The model under review builds one solid part; all positions refer to its coordinate system, in mm. Give positions to 0.01 mm unless a question says otherwise; leave off trailing zeros. Loops run counter-clockwise (first coordinate to the right, second up) from the corner with the lowest first, then second, coordinate; pieces in that order, holes last. Notation, with made-up numbers: M -30.75,0 L -11.75,0 A21 ccw -11.75,8 Z; hole C 18.5,77 d1. An arc over 180 degrees is marked long. Return JSON: item names as keys, results as strings.
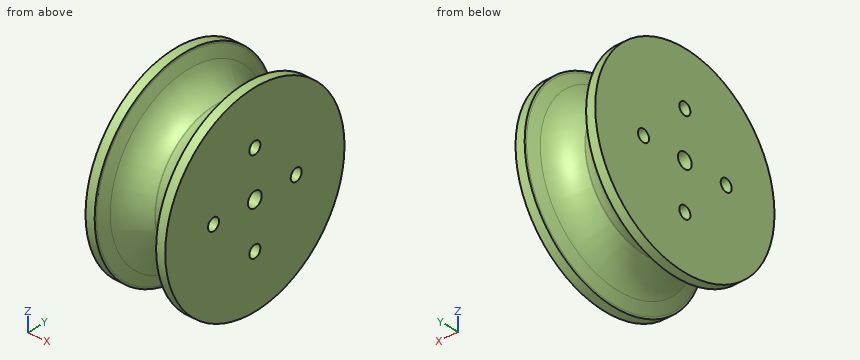
```python
from build123d import *

# Parameters (mm, degrees)
SKETCH1_W          = 3
SKETCH1_H          = 30
SKETCH2_R          = 2
CUT_EXTRUDE1_DEPTH = 31


with BuildPart() as part:
    # Sketch1 → Revolve1 (revolve)
    with BuildSketch(Plane.XY):
        with BuildLine():
            ThreePointArc((0.101961368, 31.893841841), (0, 31.900056883), (-0.101961368, 31.893841841))
            ThreePointArc((-0.101961368, 31.893841841), (-5.309821172, 29.73045951), (-8.646594366, 25.184255434))
            Line((-8.646594366, 25.184255434), (-9.965363022, 21.693397226))
            ThreePointArc((-9.965363022, 21.693397226), (-10.046395323, 21.401631123), (-10.073702174, 21.100055213))
            Line((-10.073702174, 21.100055213), (-10.073702174, 51.100055213))
            Line((-10.073702174, 51.100055213), (10.073702174, 51.100055213))
            Line((10.073702174, 51.100055213), (10.073702174, 21.100055213))
            ThreePointArc((10.073702174, 21.100055213), (10.046395323, 21.401631123), (9.965363022, 21.693397226))
            Line((9.965363022, 21.693397226), (8.646594366, 25.184255434))
            ThreePointArc((8.646594366, 25.184255434), (5.309821172, 29.73045951), (0.101961368, 31.893841841))
        make_face()
        with Locations((-11.573702174, 36.100055213)):
            Rectangle(SKETCH1_W, SKETCH1_H)
        with Locations((11.573702174, 36.100055213)):
            Rectangle(SKETCH1_W, SKETCH1_H)
    revolve(axis=Axis((-31.343058989, 53.600055213, 0), (1, 0, 0)))

    # Sketch2 → Cut-Extrude1 (cut)
    with BuildSketch(Plane.ZY.offset(13.073702174)):
        with Locations((0, 68.600055213)):
            Circle(SKETCH2_R)
        with Locations((15, 53.600055213)):
            Circle(SKETCH2_R)
        with Locations((0, 38.600055213)):
            Circle(SKETCH2_R)
        with Locations((-15, 53.600055213)):
            Circle(SKETCH2_R)
    extrude(amount=-CUT_EXTRUDE1_DEPTH, mode=Mode.SUBTRACT)


solid = part.part
```
1) Wall thickness on L1, parallel to Y at x = 3.75, z = 0; L2, parallel to Z at x = -11.25, y = 47.5; L3, parallel to Y at x = 2, z = -16: over which ranges is each line inside the solid? List them lowest first. Write a range as from..to.
From the geometry:
{"L1": "30.75..36.6, 40.6..51.1, 56.1..66.6, 70.6..76.45", "L2": "-31.92..31.92", "L3": "38.33..51.87, 55.33..68.87"}
2) Insertion check: pin 1 (8 mm diameter, centred on x = 8.5, z = -8.5, fed in from -Y); pin 2 (2 mm diameter, centred on x = 9.5, y = 68.5, fed in from -Z); pin 3 (4 mm diameter, centred on x = -10, y = 63.5, fed in from +Z). Each pin has a flat end and moves straight along its axis. Give the tip position at first contact, or say it passes through.
From the geometry:
{"pin 1": "y = 21.46", "pin 2": "z = -29.29", "pin 3": "z = 31.52"}
3) Consider section B-B on x = 5.5. Write out the cut boundary in (y, z), then the cut area to 3 significant figures.
From the geometry:
{"outline": "C 53.6,0 d48.05; hole C 38.6,0 d4; hole C 53.6,0 d5; hole C 53.6,-15 d4; hole C 53.6,15 d4; hole C 68.6,0 d4", "area": "1,740 mm²"}
4) Consider section C-C on x = -1.25. Write out the cut boundary in (y, z).
From the geometry:
{"outline": "C 53.6,0 d43.82; hole C 38.6,0 d4; hole C 53.6,0 d5; hole C 53.6,-15 d4; hole C 53.6,15 d4; hole C 68.6,0 d4"}
5) Consider section A-A on z = 0. Count the separate pieces of the cut face and the enclosed holes in it, then the cut area to 3 significant figures.
From the geometry:
{"separate pieces": "4", "enclosed holes": "0", "area": "1,040 mm²"}
